Source: CAD feature listing. Evaluate the final solid. Frame: model axes, mm. Coordinates: 2 decimals unless noted, no trailing zeros. Write each loop counter-clockwise with the first axis right and the second up, starting at its lowest first coordinate (ties: lowest second). Pieces come first, ordered by that corner, then holes. Notation, with made-up numbers: (79.25, 38.5) - (136.25, 38.5) arc R31 cw to (136.25, 68.5) - close; hole circle Ø10 at (-32.5, 32.5). An arc over 180 degrees is marked (long way). One line per question, with ' | ' between items.
from build123d import *

# Parameters (mm, degrees)
SKETCH1_R                                  = 96.266
BOSS_EXTRUDE1_DEPTH                        = 31.75
SKETCH2_R                                  = 94.996
CUT_EXTRUDE1_DEPTH                         = 30.48
F_23_64_0_35938_DIAMETER_HOLE1_D           = 9.128252
F_23_64_0_35938_DIAMETER_HOLE1_ON_FACE_2_D = 9.128252
SKETCH5_R                                  = 3.81
CUT_EXTRUDE2_DEPTH                         = 22.86


with BuildPart() as part:
    # Sketch1 → Boss-Extrude1 (new body)
    with BuildSketch(Plane(origin=(0, 0, 0), x_dir=(1, 0, 0), z_dir=(0, 1, 0))):
        with Locations(Location((0, 0, 0), (0, 0, 270))):
            Circle(SKETCH1_R)
    extrude(amount=BOSS_EXTRUDE1_DEPTH)

    # Sketch2 → Cut-Extrude1 (cut)
    with BuildSketch(Plane.XZ):
        with Locations(Location((0, 0, 0), (0, 0, 270))):
            Circle(SKETCH2_R)
    extrude(amount=-CUT_EXTRUDE1_DEPTH, mode=Mode.SUBTRACT)

    # 23/64 (0.35938) Diameter Hole1 (through all)
    with Locations(Plane(origin=(1.163e-06, 31.75, -2.517e-06), x_dir=(0, 0, 1), z_dir=(0, 1, 0))):
        with Locations((0, 0)):
            Hole(F_23_64_0_35938_DIAMETER_HOLE1_D / 2)

    # 23/64 (0.35938) Diameter Hole1 on face 2 (through all)
    with Locations(Plane.ZX):
        with Locations((0, 0)):
            Hole(F_23_64_0_35938_DIAMETER_HOLE1_ON_FACE_2_D / 2)

    # Sketch5 → Cut-Extrude2 (cut)
    with BuildSketch(Plane(origin=(0, 31.75, 0), x_dir=(1, 0, 0), z_dir=(0, 1, 0))):
        with Locations(Location((72.382124837, 0, 0), (0, 0, 270))):
            Circle(SKETCH5_R)
        with Locations(Location((36.191062419, 62.684758889, 0), (0, 0, 270))):
            Circle(SKETCH5_R)
        with Locations(Location((-36.191062419, 62.684758889, 0), (0, 0, 270))):
            Circle(SKETCH5_R)
        with Locations(Location((-72.382124837, 0, 0), (0, 0, 270))):
            Circle(SKETCH5_R)
        with Locations(Location((-36.191062419, -62.684758889, 0), (0, 0, 270))):
            Circle(SKETCH5_R)
        with Locations(Location((36.191062419, -62.684758889, 0), (0, 0, 270))):
            Circle(SKETCH5_R)
    extrude(amount=-CUT_EXTRUDE2_DEPTH, mode=Mode.SUBTRACT)


solid = part.part
Item 1: Mould query, pull axis X, two halves, no side actions, for faces 1 (the face through (-93.977, 15.653, -20.869)), 2 (the face through (1, 31.75, 20)), 3 (the face through (-20, 30.48, 1)), 4 (the face through (28.53, 15.03, -90.61)). Classes: pulls with the +X half, pulls with the -X half, needs draft (parallel to the pull), parting line crosses it, or undercut.
Check sheet entries:
face 1: parting line crosses it | face 2: needs draft | face 3: undercut | face 4: undercut
Item 2: Cut plane A-A on z = 0. Return loops of the section in (x, y), and give its area (3 significant figures).
Check sheet entries:
outline: (-96.27, 0) - (-95, 0) - (-95, 30.48) - (-76.19, 30.48) - (-76.19, 31.75) - (-96.27, 31.75) - close; (-68.57, 30.48) - (-4.56, 30.48) - (-4.56, 31.75) - (-68.57, 31.75) - close; (4.56, 30.48) - (68.57, 30.48) - (68.57, 31.75) - (4.56, 31.75) - close; (76.19, 30.48) - (95, 30.48) - (95, 0) - (96.27, 0) - (96.27, 31.75) - (76.19, 31.75) - close | area: 291 mm²
Item 3: Cut plane B-B on z = 63.5. Return loops of the section in (x, y), and give its area (3 significant figures).
Check sheet entries:
outline: (-72.35, 0) - (-70.65, 0) - (-70.65, 30.48) - (-39.91, 30.48) - (-39.91, 31.75) - (-72.35, 31.75) - close; (-32.47, 30.48) - (32.47, 30.48) - (32.47, 31.75) - (-32.47, 31.75) - close; (39.91, 30.48) - (70.65, 30.48) - (70.65, 0) - (72.35, 0) - (72.35, 31.75) - (39.91, 31.75) - close | area: 268 mm²
Item 4: Cut plane D-D on z = -21.5. Return loops of the section in (x, y), and give its area (3 significant figures).
Check sheet entries:
outline: (-93.83, 0) - (-92.53, 0) - (-92.53, 30.48) - (92.53, 30.48) - (92.53, 0) - (93.83, 0) - (93.83, 31.75) - (-93.83, 31.75) - close | area: 318 mm²
Item 5: Pin query (flat end, axial travel): pin 1 Ø4 at (x, y) = (-8, 13) entering from +Z; pin 2 Ø1.5 at (x, z) = (30, -27.5) entering from -Y; pin 3 Ø12 at (x, y) = (-46.5, 4) entering from +Z. Return the tip coordinate at first contact, or that it passes through.
Check sheet entries:
pin 1: z = 96.08 | pin 2: y = 30.48 | pin 3: z = 87.33
Item 6: Ray query, line 1 along X through (y, z) = (31.1, 0); line 2 along Z through (x, y) = (2.5, 19); line 3 along Y through (x, z) = (-62.5, -34.5). Return the intervals inside material, ascending. Write a range as [from, to].
Check sheet entries:
line 1: [-96.27, -76.19], [-68.57, -4.56], [4.56, 68.57], [76.19, 96.27] | line 2: [-96.23, -94.96], [94.96, 96.23] | line 3: [30.48, 31.75]
Item 7: Cut plane C-C on x = -55. Return loops of the section in (y, z).
Check sheet entries:
outline: (0, -79.01) - (31.75, -79.01) - (31.75, 79.01) - (0, 79.01) - (0, 77.45) - (30.48, 77.45) - (30.48, -77.45) - (0, -77.45) - close
